Autodesk Inventor part; units mm, degrees
ref_plane "YZ Plane" through (0, 0, 0) normal (1, 0, 0) x (0, 1, 0)
ref_plane "XZ Plane" through (0, 0, 0) normal (0, 1, 0) x (-1, 0, 0)
ref_plane "XY Plane" through (0, 0, 0) normal (0, 0, 1) x (1, 0, 0)
ref_plane "Work Plane1" through (0, 0, 0) normal (0, 0, 1) x (1, 0, 0)
sketch "Sketch1" plane through (0, 0, 0) normal (0, 0, 1) x (1, 0, 0)
  line L0 (0, 0) -> (30, 0)
  line L1 (0, 0) -> (0, -6)
  line L2 (30, -6) -> (0, -6)
  line L3 (30, 0) -> (30, -6)
  line L4 (60, 0) -> (90, 0)
  line L5 (60, 0) -> (60, -6)
  line L6 (90, -6) -> (60, -6)
  line L7 (90, 0) -> (90, -6)
  line L8 (120, 0) -> (150, 0)
  line L9 (120, 0) -> (120, -6)
  line L10 (150, -6) -> (120, -6)
  line L11 (150, 0) -> (150, -6)
  line L12 (30, 0) -> (60, 0)
  line L13 (90, 0) -> (120, 0)
  line L14 (150, 0) -> (164.8734, 0)
  line L15 (0, 0) -> (-14.8734, 0)
  line L16 (-20.8734, -6) -> (0, -6)
  line L17 (150, -6) -> (170.8734, -6)
  line L18 (0, 0) -> (0, -6)
  line L19 (30, -6) -> (0, -6)
  line L20 (30, -6) -> (30, 0)
  line L21 (60, 0) -> (60, -6)
  line L22 (90, -6) -> (60, -6)
  line L23 (90, -6) -> (90, 0)
  line L24 (120, 0) -> (120, -6)
  line L25 (120, -6) -> (150, -6)
  line L26 (150, 0) -> (150, -6)
  line L27 (164.8734, 0) -> (164.8734, 100)
  line L28 (-14.8734, 0) -> (-14.8734, 100)
  line L29 (-14.8734, 100) -> (164.8734, 100)
  line L30 (164.8734, 20) -> (170.8734, 20)
  line L31 (170.8734, 20) -> (170.8734, 40)
  line L32 (170.8734, 40) -> (164.8734, 40)
  line L33 (164.8734, 40) -> (164.8734, 20)
  line L34 (164.8734, 60) -> (170.8734, 60)
  line L35 (170.8734, 60) -> (170.8734, 80)
  line L36 (170.8734, 80) -> (164.8734, 80)
  line L37 (164.8734, 80) -> (164.8734, 60)
  line L38 (-14.8734, 80) -> (-20.8734, 80)
  line L39 (-20.8734, 80) -> (-20.8734, 60)
  line L40 (-20.8734, 60) -> (-14.8734, 60)
  line L41 (-14.8734, 60) -> (-14.8734, 80)
  line L42 (-14.8734, 20) -> (-20.8734, 20)
  line L43 (-20.8734, 20) -> (-20.8734, 40)
  line L44 (-20.8734, 40) -> (-14.8734, 40)
  line L45 (-14.8734, 40) -> (-14.8734, 20)
  dimension "d0" = 6
  dimension "d1" = 6
  dimension "d2" = 100
  dimension "d3" = 100
  dimension "d5" = 20
  dimension "d6" = 20
  dimension "d7" = 20
  dimension "d8" = 6
extrude "Plate1" add sketch "Sketch1" along normal blind 6
equation "\"d6\" = d5"
equation "\"d7\" = d5"
equation "\"d4\" = Thickness"
equation "\"BendRadius\" = Thickness"
equation "\"BendReliefWidth\" = Thickness"
equation "\"BendReliefDepth\" = 0.5 * Thickness"
equation "\"CornerReliefSize\" = 4 * Thickness"
equation "\"MinimumRemnant\" = 2 * Thickness"
equation "\"TransitionRadius\" = BendRadius"
equation "\"JacobiRadiusSize\" = BendRadius"
equation "\"GapSize\" = Thickness"
properties part number "zijkant2 electronica" material "Wood (Birch)"
Check sheet for the modelled part. Datum: model origin and axes. Units: mm. A direction names the side the tool comes from. Coordinates: 2 decimals unless noted, no trailing zeros. Loops run counter-clockwise (first coordinate to the right, second up) from the corner with the lowest first, then second, coordinate; pieces in that order, holes last. Notation, with made-up numbers: (-4.5, 14) -> (52.5, 14) arc R13 ccw to (52.5, 20) -> close; hole circle Ø2 at (52, -20.5). An arc over 180 degrees is marked (long way). Write item = value, one per line. Start each with the question number.
1. Material ranges on line 1 (Y direction, x = -7, z = 0.95); line 2 (X direction, y = 57.5, z = 3.65), recorded low to high.
2. Draft check along Y on faces 5 (the flat face through (168, 80, 3)), 6 (the flat face through (-14.873, 50, 3)), 7 (the flat face through (157, 0, 3)). Enter one of: released by +Y, released by -Y, zero draft, split by the parting line, or undercut.
3. Section check C-C on y = 48.5. Record the cut outline in (x, z), then the cut area to 3 significant figures.
4. Depth check by flat-ended pin: P1, Ø1.8, axis at y = 46.5, z = 2.5, coming from the -X side; P2, Ø1.5, axis at x = 81, y = 10.5, coming from the -Z side; P3, Ø2, axis at x = 107, z = 3.5, coming from the -Y side; P4, Ø3, axis at y = -3.5, z = 2.5, coming from the +X side. Enter the tip coordinate at first touch or a pass-through.
5. Tool access check on faces 1 (the flat face through (120, -3, 3)), 2 (the flat face through (-18, 20, 3)), 3 (the flat face through (164.873, 10, 3)), 4 (the flat face through (-18, 40, 3)). Record the directions out of +Z, -Z, +X, -X, +Y, -Y that give a thin tool (end or side, any length) a straight path to the whole face; none if there is none.
6. Section check B-B on x = 37.5. Record the cut outline in (y, z), then the cut area to 3 significant figures.
Responses:
q1.line_1 = 0 to 100
q1.line_2 = -14.87 to 164.87
q2.face_5 = released by +Y
q2.face_6 = undercut
q2.face_7 = released by -Y
q3.outline = (-14.87, 0) -> (164.87, 0) -> (164.87, 6) -> (-14.87, 6) -> close
q3.area = 1,080 mm2
q4.P1 = -14.87
q4.P2 = 0
q4.P3 = 0
q4.P4 = 150
q5.face_1 = +Z, -Z, -Y
q5.face_2 = +Z, -Z, -X, -Y
q5.face_3 = +Z, -Z, +X, -Y
q5.face_4 = +Z, -Z, -X
q6.outline = (0, 0) -> (100, 0) -> (100, 6) -> (0, 6) -> close
q6.area = 600 mm2
